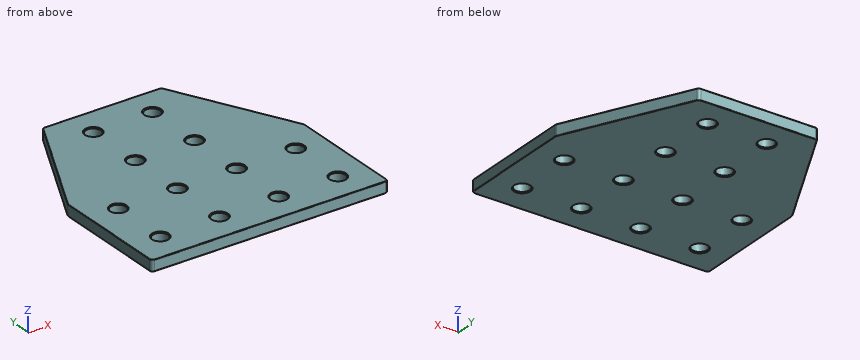
```python
from build123d import *

# Parameters (mm, degrees)
BOSS_EXTRUDE1_START = 2.3876
SKETCH3_R           = 3.2639
BOSS_EXTRUDE1_DEPTH = 4.7752
FILLET1_R           = 1.27
CHAMFER1_SIZE       = 0.381
FILLET2_R           = 0.254


with BuildPart() as part:
    # Sketch3 → Boss-Extrude1 (new body)
    with BuildSketch(Plane.XY.offset(BOSS_EXTRUDE1_START)):
        Polygon((25.4, 50.8), (50.8, 0), (50.8, -50.8), (-50.8, -50.8), (-50.8, 0), (-25.4, 50.8), align=None)
        with Locations((-38.1, -38.1)):
            Circle(SKETCH3_R, mode=Mode.SUBTRACT)
        with Locations((-12.7, -38.1)):
            Circle(SKETCH3_R, mode=Mode.SUBTRACT)
        with Locations((12.7, -38.1)):
            Circle(SKETCH3_R, mode=Mode.SUBTRACT)
        with Locations((38.1, -38.1)):
            Circle(SKETCH3_R, mode=Mode.SUBTRACT)
        with Locations((-12.7, -12.7)):
            Circle(SKETCH3_R, mode=Mode.SUBTRACT)
        with Locations((12.7, -12.7)):
            Circle(SKETCH3_R, mode=Mode.SUBTRACT)
        with Locations((38.1, -12.7)):
            Circle(SKETCH3_R, mode=Mode.SUBTRACT)
        with Locations((-12.7, 12.7)):
            Circle(SKETCH3_R, mode=Mode.SUBTRACT)
        with Locations((12.7, 12.7)):
            Circle(SKETCH3_R, mode=Mode.SUBTRACT)
        with Locations((-12.7, 38.1)):
            Circle(SKETCH3_R, mode=Mode.SUBTRACT)
        with Locations((12.7, 38.1)):
            Circle(SKETCH3_R, mode=Mode.SUBTRACT)
        with Locations((-38.1, -12.7)):
            Circle(SKETCH3_R, mode=Mode.SUBTRACT)
    extrude(amount=-BOSS_EXTRUDE1_DEPTH)

    # Fillet1
    fillet1_edges = [part.edges().sort_by_distance(p)[0] for p in [
        (25.4, 50.8, 0),
        (50.8, 0, 0),
        (50.8, -50.8, 0),
        (-50.8, -50.8, 0),
        (-50.8, 0, 0),
        (-25.4, 50.8, 0),
    ]]
    fillet(fillet1_edges, radius=FILLET1_R)

    # Chamfer1
    chamfer1_edges = [part.edges().sort_by_distance(p)[0] for p in [
        (-41.3639, -38.1, -2.3876),
        (-41.3639, -38.1, 2.3876),
        (-15.9639, -38.1, -2.3876),
        (-15.9639, -38.1, 2.3876),
        (9.4361, -38.1, -2.3876),
        (9.4361, -38.1, 2.3876),
        (34.8361, -38.1, -2.3876),
        (34.8361, -38.1, 2.3876),
        (-15.9639, -12.7, -2.3876),
        (-15.9639, -12.7, 2.3876),
        (9.4361, -12.7, -2.3876),
        (9.4361, -12.7, 2.3876),
        (34.8361, -12.7, -2.3876),
        (34.8361, -12.7, 2.3876),
        (-15.9639, 12.7, -2.3876),
        (-15.9639, 12.7, 2.3876),
        (9.4361, 12.7, -2.3876),
        (9.4361, 12.7, 2.3876),
        (-15.9639, 38.1, -2.3876),
        (-15.9639, 38.1, 2.3876),
        (9.4361, 38.1, -2.3876),
        (9.4361, 38.1, 2.3876),
        (-41.3639, -12.7, -2.3876),
        (-41.3639, -12.7, 2.3876),
    ]]
    chamfer(chamfer1_edges, length=CHAMFER1_SIZE)

    # Fillet2
    fillet2_edges = [part.edges().sort_by_distance(p)[0] for p in [
        (0, 50.8, 2.3876),
        (0, 50.8, -2.3876),
        (-38.20847095, 25.183058101, 2.3876),
        (-50.8, -24.914903166, 2.3876),
        (0, -50.8, 2.3876),
        (50.8, -24.914903166, 2.3876),
        (38.20847095, 25.183058101, 2.3876),
        (50.766026217, -0.008020122, 2.3876),
        (50.428025612, -50.428025612, 2.3876),
        (25.282775347, 50.610326527, 2.3876),
        (-50.428025612, -50.428025612, 2.3876),
        (-50.766026217, -0.008020122, 2.3876),
        (-25.282775347, 50.610326527, 2.3876),
        (-38.20847095, 25.183058101, -2.3876),
        (38.20847095, 25.183058101, -2.3876),
        (50.8, -24.914903166, -2.3876),
        (0, -50.8, -2.3876),
        (-50.8, -24.914903166, -2.3876),
        (50.766026217, -0.008020122, -2.3876),
        (50.428025612, -50.428025612, -2.3876),
        (25.282775347, 50.610326527, -2.3876),
        (-50.428025612, -50.428025612, -2.3876),
        (-50.766026217, -0.008020122, -2.3876),
        (-25.282775347, 50.610326527, -2.3876),
    ]]
    fillet(fillet2_edges, radius=FILLET2_R)


solid = part.part
```
Build history of the part. All positions in model axes, mm. Give positions to 0.01 mm unless a question says otherwise; leave off trailing zeros. Return JSON: item names as keys, results as strings.
Q1. Flat gauge pins, fed straight in: pin 1 (7.5 mm diameter, centred on x = -38.1, y = -38.1, fed in from +Z); pin 2 (5 mm diameter, centred on x = -12.7, y = 12.7, fed in from -Z). Where does each tip first touch, or does it go through?
Answer list:
{"pin 1": "stops at z = 2.39", "pin 2": "passes through"}
Q2. Wall check: probe 1 along Y at (x, z) = (-12.7, -0.75); probe 2 along Y at (x, z) = (-37, -1.2); probe 3 along Y at (x, z) = (38.1, 0.65). Give the ranges that are in metal, low to high. Write a range as from..to.
Answer list:
{"probe 1": "y = -50.8..-41.36, -34.84..-15.96, -9.44..9.44, 15.96..34.84, 41.36..50.8", "probe 2": "y = -50.8..-41.17, -35.03..-15.77, -9.63..27.6", "probe 3": "y = -50.8..-41.36, -34.84..-15.96, -9.44..25.4"}
Q3. Band-saw the part on A-A (z = -0.9). Count the separate pieces of the cut face and the enclosed holes in it, then the cut area to 3 significant figures.
Answer list:
{"separate pieces": "1", "enclosed holes": "12", "area": "8,630 mm^2"}
